Read the model definition and answer for the solid it produces. Units are mm, in the model's axes. Face numbers are marked on the shaded views. A direction names the side the tool comes from. Give positions to 0.01 mm unless a question says otherwise; leave off trailing zeros. Order: outer loops, then holes, each group sorted by start corner. A loop starts at its lowest first (then second) coordinate and runs counter-clockwise, first axis right, second up. Notation, with made-up numbers: (60.25, 84.5) - (75.25, 84.5) arc R8 ccw to (75.25, 97.5) - close; hole circle Ø5 at (55.5, 31). An arc over 180 degrees is marked (long way). Use a Markdown table: item, result. Add a question column.
1. Which of the six approach directions +Z, -Z, +X, -X, +Y, -Y give full straight-line access (tool end or side, diameter ignored) to the marked faces 4, 5, 6 and 7?
2. A cutting plane is placed at A-A on y = -12. Determine the outline of the cut face in (x, z), and give its area (3 significant figures).
3. A cutting plane is placed at B-B on y = 1. Determine the outline of the cut face in (x, z), and give its area (3 significant figures).
4. Consider L1, parallel to X at y = -10.5, z = -8.5; L2, parallel to Y at x = 8.75, z = -8; L3, parallel to Y at x = 5, z = -7.75. Determine where each line is inside the solid, lowest interval first.
5. For a pull along Y with two mould halves and no side action, classify the marked faces 1, 2 and 3 as released by +Y, released by -Y, zero draft, split by the parting line, or undercut.
6. Flat-ended cylindrical pins translate along their axes: P1, Ø8, axis at y = 1, z = -8, coming from the -X side; P2, Ø2, axis at y = -8, z = -10, coming from the +X side; P3, Ø6.5, axis at x = -23, z = -6, coming from the +Y side; P4, Ø4, axis at x = -9.5, y = -6.5, coming from the +Z side. Find the tip coordinate at first contact, or state that the pin passes through.
7. A cutting plane is placed at D-D on z = -2.25. Determine the outline of the cut face in (x, y).
8. A cutting plane is placed at C-C on y = 7. Determine the outline of the cut face in (x, z), and give its area (3 significant figures).
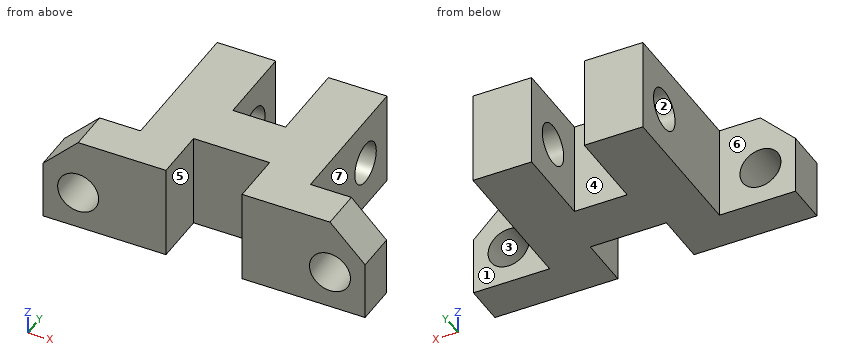
```python
from build123d import *

# Parameters (mm, degrees)
BOSS_EXTRUDE1_DEPTH     = 16
CUT_EXTRUDE1_DEPTH      = 49.414873748
CUT_EXTRUDE1_DEPTH_BACK = 49.414873748
SKETCH2_R               = 3.5
CHAMFER1_SIZE           = 6
CHAMFER2_SIZE           = 6
CUT_EXTRUDE2_DEPTH      = 41.462946012
CUT_EXTRUDE2_DEPTH_BACK = 16
SKETCH6_R               = 3.5
SKETCH6_3_R             = 3.5
CUT_EXTRUDE3_DEPTH      = 16


with BuildPart() as part:
    # Sketch1 → Boss-Extrude1 (new body)
    with BuildSketch(Plane.XY):
        Polygon((4.5, 0), (-4.5, 0), (-4.5, 14), (-14.5, 14), (-14.5, -11), (-27.5, -11), (-27.5, -18), (-6.5, -18), (-6.5, -9), (6.5, -9), (6.5, -18), (27.5, -18), (27.5, -11), (14.5, -11), (14.5, 14), (4.5, 14), align=None)
    extrude(amount=-BOSS_EXTRUDE1_DEPTH)

    # Sketch2 → Cut-Extrude1 (cut, two sides: drawn at the far end of the back side and taken through both)
    with BuildSketch(Plane(origin=(14.5, 0, 0), x_dir=(0, 0, -1), z_dir=(1, 0, 0)).offset(-CUT_EXTRUDE1_DEPTH_BACK)):
        with Locations((8, 7)):
            Circle(SKETCH2_R)
    extrude(amount=CUT_EXTRUDE1_DEPTH + CUT_EXTRUDE1_DEPTH_BACK, mode=Mode.SUBTRACT)

    # Chamfer1
    chamfer1_edges = [part.edges().sort_by_distance(p)[0] for p in [
        (-27.5, -14.5, 0),
    ]]
    chamfer(chamfer1_edges, length=CHAMFER1_SIZE)

    # Chamfer2
    chamfer2_edges = [part.edges().sort_by_distance(p)[0] for p in [
        (27.5, -14.5, 0),
    ]]
    chamfer(chamfer2_edges, length=CHAMFER2_SIZE)

    # Sketch6 → Cut-Extrude2 (cut, two sides: drawn at the far end of the back side and taken through both)
    with BuildSketch(Plane(origin=(0, -11, 0), x_dir=(1, 0, 0), z_dir=(0, 1, 0)).offset(-CUT_EXTRUDE2_DEPTH_BACK)):
        with Locations(Location((-21.5, 9.5, 0), (0, 0, 90))):
            Circle(SKETCH6_R)
    extrude(amount=CUT_EXTRUDE2_DEPTH + CUT_EXTRUDE2_DEPTH_BACK, mode=Mode.SUBTRACT)

    # Sketch6_3 → Cut-Extrude3 (cut)
    with BuildSketch(Plane(origin=(0, -11, 0), x_dir=(1, 0, 0), z_dir=(0, 1, 0))):
        with Locations(Location((21.5, 9.5, 0), (0, 0, 180))):
            Circle(SKETCH6_3_R)
    extrude(amount=-CUT_EXTRUDE3_DEPTH, mode=Mode.SUBTRACT)


solid = part.part
```
Output values:
| question | item | result |
|---|---|---|
| 1 | face 4 | +Z, -Z, +Y |
| 1 | face 5 | +Z, -Z, -Y |
| 1 | face 6 | +Z, -Z, -X, +Y |
| 1 | face 7 | +Z, -Z, +X, +Y |
| 2 | outline | (-27.5, -16) - (-6.5, -16) - (-6.5, 0) - (-21.5, 0) - (-27.5, -6) - close; (6.5, -16) - (27.5, -16) - (27.5, -6) - (21.5, 0) - (6.5, 0) - close; hole circle Ø7 at (-21.5, -9.5); hole circle Ø7 at (21.5, -9.5) |
| 2 | area | 559 mm² |
| 3 | outline | (-14.5, -16) - (-4.5, -16) - (-4.5, 0) - (-14.5, 0) - close; (4.5, -16) - (14.5, -16) - (14.5, 0) - (4.5, 0) - close |
| 3 | area | 320 mm² |
| 4 | L1 | -14.5 to -6.5, 6.5 to 14.5 |
| 4 | L2 | -18 to 3.5, 10.5 to 14 |
| 4 | L3 | -9 to 3.51, 10.49 to 14 |
| 5 | face 1 | released by +Y |
| 5 | face 2 | undercut |
| 5 | face 3 | zero draft |
| 6 | P1 | x = -14.5 |
| 6 | P2 | x = 14.5 |
| 6 | P3 | y = -11 |
| 6 | P4 | z = 0 |
| 7 | outline | (-23.75, -18) - (-6.5, -18) - (-6.5, -9) - (6.5, -9) - (6.5, -18) - (23.75, -18) - (23.75, -11) - (14.5, -11) - (14.5, 14) - (4.5, 14) - (4.5, 0) - (-4.5, 0) - (-4.5, 14) - (-14.5, 14) - (-14.5, -11) - (-23.75, -11) - close |
| 8 | outline | (-14.5, -16) - (-4.5, -16) - (-4.5, -11.5) - (-14.5, -11.5) - close; (-14.5, -4.5) - (-4.5, -4.5) - (-4.5, 0) - (-14.5, 0) - close; (4.5, -16) - (14.5, -16) - (14.5, -11.5) - (4.5, -11.5) - close; (4.5, -4.5) - (14.5, -4.5) - (14.5, 0) - (4.5, 0) - close |
| 8 | area | 180 mm² |
